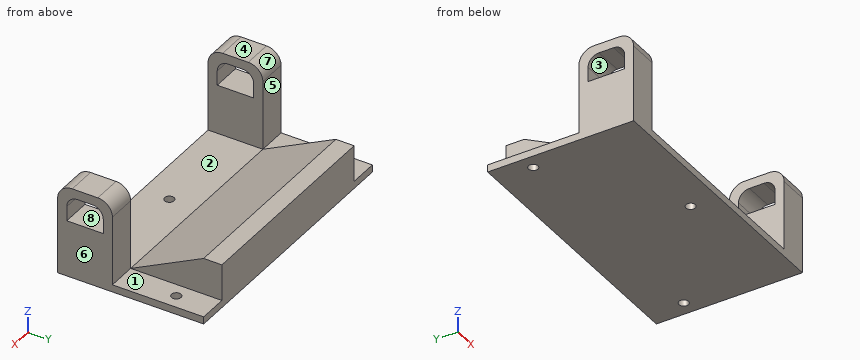
Autodesk Fusion 360 part; units mm, degrees
sketch "Sketch1" plane through (0, 0, 0) normal (0, 0, 1) x (1, 0, 0)
  line L0 (0, 0) -> (74, 0)
  line L1 (74, 0) -> (74, 40)
  line L2 (74, 40) -> (0, 40)
  line L3 (0, 40) -> (0, 0)
  line L4 (0, 0) -> (74, 0)
  line L5 (74, 0) -> (74, 15)
  line L6 (74, 15) -> (0, 15)
  line L7 (0, 15) -> (0, 0)
  line L8 (0, 15) -> (8, 15)
  line L9 (8, 15) -> (8, 0)
  line L10 (8, 0) -> (0, 0)
  line L11 (0, 0) -> (0, 15)
  line L12 (74, 15) -> (66, 15)
  line L13 (66, 15) -> (66, 0)
  line L14 (66, 0) -> (74, 0)
  line L15 (74, 0) -> (74, 15)
  line L16 (8, 15) -> (66, 15)
  line L17 (66, 15) -> (66, 40)
  line L18 (66, 40) -> (8, 40)
  line L19 (8, 40) -> (8, 15)
  circle A0 centre (4, 30) radius 1.3
  circle A1 centre (70, 30) radius 1.3
  circle A2 centre (37, 7.5) radius 1.3
  dimension "d1" = 74
  dimension "d2" = 40
  dimension "d3" = 15
  dimension "d6" = 8
  dimension "d7" = 8
  dimension "d16" = 2.6
  dimension "d17" = 4
  dimension "d18" = 2.6
  dimension "d19" = 4
  dimension "d20" = 10
  dimension "d21" = 10
  dimension "d22" = 2.6
  dimension "d23" = 7.5
  dimension "d24" = 37
  dimension "d35" = 8
extrude "Extrude1" add sketch "Sketch1" along normal blind 2 contours L0 L3 L4 L6 L7 L8 L9 L10 L11 | L0 L4 L6 L9 L13 L16 | L2 L3 L6 L8 L19 | L0 L1 L4 L5 L6 L12 L13 L14 L15 | L2 L6 L16 L17 L18 L19 | L1 L2 L6 L12 L17 | A0 | A1 | A2
extrude "Extrude5" add sketch "Sketch1" along normal blind 12 contours L2 L6 L16 L17 L18 L19
chamfer "Chamfer1" distance 20 distance2 10 1 edges at (37, 15, 12) measured on face at (27.3333, 31.6667, 12)
extrude "Extrude2" add sketch "Sketch1" along normal blind 25 contours L0 L3 L4 L6 L7 L8 L9 L10 L11 | L0 L1 L4 L5 L6 L12 L13 L14 L15
sketch "Sketch2" plane through (74, 0, 0) normal (1, 0, 0) x (0, 1, 0)
  line L0 (0, 0) -> (40, 0)
  line L1 (40, 0) -> (40, 2)
  line L2 (40, 2) -> (15, 2)
  line L3 (15, 2) -> (15, 25)
  line L4 (15, 25) -> (0, 25)
  line L5 (0, 25) -> (0, 0)
  line L6 (2.5, 22.5) -> (12.5, 22.5)
  line L7 (12.5, 22.5) -> (12.5, 15.5)
  line L8 (12.5, 15.5) -> (2.5, 15.5)
  line L9 (2.5, 15.5) -> (2.5, 22.5)
  dimension "d10" = 2.5
  dimension "d11" = 2.5
  dimension "d12" = 2.5
  dimension "d13" = 7
extrude "Extrude3" cut sketch "Sketch2" against normal blind 100 contours L6 L7 L8 L9
extrude "Extrude4" cut sketch "Sketch1" along normal blind 10 contours A0 | A1 | A2
fillet "Fillet1" radius 3 4 edges at (70, 12.5, 22.5) (4, 12.5, 22.5) (70, 2.5, 22.5) (4, 2.5, 22.5)
fillet "Fillet2" radius 4 4 edges at (4, 15, 25) (4, 0, 25) (70, 0, 25) (70, 15, 25)
Design review of the part built by this model. Coordinates are the model's own, in mm. Face numbers are marked on the shaded views. A direction names the side the tool comes from. Coordinates: 2 decimals unless noted, no trailing zeros. Write each loop counter-clockwise with the first axis right and the second up, starting at its lowest first coordinate (ties: lowest second). Pieces come first, ordered by that corner, then holes. Notation, with made-up numbers: (-4.5, -26) - (45.5, -26) arc R17 ccw to (45.5, 6) - close; hole circle Ø2 at (38, 21). An arc over 180 degrees is marked (long way). One line per item, written item: value.
1) Add section B-B (x = 4). State the section outline as (y, z) points.
Answer sheet:
outline: (0, 0) - (28.7, 0) - (28.7, 2) - (15, 2) - (15, 21) arc R4 ccw to (11, 25) - (4, 25) arc R4 ccw to (0, 21) - close; (31.3, 0) - (40, 0) - (40, 2) - (31.3, 2) - close; hole (2.5, 15.5) - (12.5, 15.5) - (12.5, 19.5) arc R3 ccw to (9.5, 22.5) - (5.5, 22.5) arc R3 ccw to (2.5, 19.5) - close
2) Mouldability with a two-part tool opening along Y and no side actions: class the marked faces 6, 7 and 8 as +Y half, -Y half, draft (parallel to the pull), parting line (faces both ways), or undercut.
Answer sheet:
face 6: draft
face 7: +Y half
face 8: undercut
3) Add section C-C (y = 7.5). State the section outline as (x, z) points.
Answer sheet:
outline: (0, 0) - (35.7, 0) - (35.7, 2) - (8, 2) - (8, 15.5) - (0, 15.5) - close; (0, 22.5) - (8, 22.5) - (8, 25) - (0, 25) - close; (38.3, 0) - (74, 0) - (74, 15.5) - (66, 15.5) - (66, 2) - (38.3, 2) - close; (66, 22.5) - (74, 22.5) - (74, 25) - (66, 25) - close
4) Insertion check: pin 1 (1 mm diameter, centred on x = 56, y = 31, fed in from +Z); pin 2 (5 mm diameter, centred on x = 44.5, y = 33.5, fed in from +Z); pin 3 (2.5 mm diameter, centred on x = 37, y = 7.5, fed in from +Z); pin 4 (2.5 mm diameter, centred on x = 69, y = 33.5, fed in from +Z). Each pin has a flat end and moves straight along its axis. Give the tip position at first contact, or say it passes through.
Answer sheet:
pin 1: stops at z = 10.25
pin 2: stops at z = 12
pin 3: passes through
pin 4: stops at z = 2
5) For the marked faces 1, 2, 3, 4 and 5, list the 3-axis set-ups (+Z, -Z, +X, -X, +Y, -Y) from which the entire face can be reached by the end or side of a thin tool; tool diameter is ignored.
Answer sheet:
face 1: +Z, +X, +Y
face 2: +Z, -Y
face 3: +X, -X
face 4: +Z, +X, -X, +Y, -Y
face 5: +Z, +X, -X, +Y
6) Add section A-A (z = 13.75). State the section outline as (x, y) points.
Answer sheet:
outline: (0, 0) - (8, 0) - (8, 15) - (0, 15) - close; (66, 0) - (74, 0) - (74, 15) - (66, 15) - close
7) To check wall thickness, follow probe 1 along X at (y, z) = (30, 1.55); probe 2 along X at (y, z) = (3, 3.5); probe 3 along Y at (x, z) = (70, 0.7). State the ranges of each line that lie inside material, in increasing order.
Answer sheet:
probe 1: x = 0 to 2.7, 5.3 to 68.7, 71.3 to 74
probe 2: x = 0 to 8, 66 to 74
probe 3: y = 0 to 28.7, 31.3 to 40
